Verification items for the finished model (mm, model axes). A direction names the side the tool comes from. Round coordinates to 2 decimals unless told otherwise and drop trailing zeros. Order: outer loops, then holes, each group sorted by start corner. A loop starts at its lowest first (then second) coordinate and runs counter-clockwise, first axis right, second up. Notation, with made-up numbers: M -5,50.25 L -1,50.25 A21 ccw -1,81.25 Z; hole C 5,35.25 d4. An arc over 180 degrees is marked long. Use CSV: the item, a comma, the result in double quotes. Start each with the question number.
Q1. Sectioned sample at A-A (z = 22.5). Enter the section's corners in (x, y).
Q2. Sectioned sample at B-B (x = 9.5). Enter the section's corners in (y, z), and give its area (3 significant figures).
Q3. Sectioned sample at C-C (x = 24.3). Enter the section's corners in (y, z).
Q4. Mould release check, pull along Y, two halves, no side actions. Record for faces 1 (the face through (-22.3, 4.78, 29.48)), 2 (the face through (8, 0, 40)), 3 (the face through (22, -1, 31)), 4 (the face through (22.3, -4.77, 29.48)): +Y half, -Y half, draft (parallel to the pull), parting line (faces both ways), or undercut.
Q5. Sectioned sample at D-D (x = 1). Enter the section's corners in (y, z).
Q6. Gauge pin test, flat ends, axial feed: pin 1 Ø4 at (y, z) = (-4.5, 12) entering from +X; pin 2 Ø8 at (x, y) = (-21.5, -7.5) entering from +Z; pin 3 Ø5 at (x, y) = (-16, 2.5) entering from +Z. Record the tip position at first contact, or that the pin passes through.
Q7. Set-up check for faces 5 (the face through (20, -0.2, 38.3)), 6 (the face through (22, 1, 31)), 7 (the face through (18, -8, 38)), 8 (the face through (20, 0, 14)): record each of +Z, -Z, +X, -X, +Y, -Y from which the full face is reachable in a straight line by a thin tool's end or side.
Q8. Scan lines: line 1 (Y direction, x = -24.3, z = 29.1); line 2 (Z direction, x = 1, y = 5.75); line 3 (X direction, y = -6.25, z = 10.5). Record each from-to range of solid material in increasing order.
Autodesk Inventor part; units mm, degrees
ref_plane "Work Plane1" through (0, 0, 28.3) normal (0, 0, 1) x (1, 0, 0)
ref_plane "YZ Plane" through (0, 0, 0) normal (1, 0, 0) x (0, 1, 0)
ref_plane "XZ Plane" through (0, 0, 0) normal (0, 1, 0) x (-1, 0, 0)
sketch "Sketch1" plane through (0, 0, 0) normal (0, 0, 1) x (1, 0, 0)
  line L0 (-20, -10) -> (20, -10)
  line L1 (20, -10) -> (20, 10)
  line L2 (20, 10) -> (-20, 10)
  line L3 (-20, 10) -> (-20, -10)
  line L4 (-20, -10) -> (20, 10) construction
  line L5 (20, -10) -> (-20, 10) construction
  point P0 (0, 0)
  dimension "d0" = 40
  dimension "d1" = 20
extrude "Extrusion1" add sketch "Sketch1" along normal blind 39
ref_plane "Work Plane1" through (0, 0, 28.3) normal (0, 0, 1) x (1, 0, 0)
sketch "Sketch2" plane through (0, 0, 28.3) normal (0, 0, 1) x (1, 0, 0)
  line L0 (20, -10) -> (-20, -10)
  line L1 (-20, -10) -> (-20, 10)
  line L2 (-20, 10) -> (20, 10)
  line L3 (20, 10) -> (20, -10)
  line L4 (-27, -10) -> (27, -10)
  line L5 (27, -10) -> (27, 10)
  line L6 (27, 10) -> (-27, 10)
  line L7 (-27, 10) -> (-27, -10)
  line L8 (-27, -10) -> (27, 10) construction
  line L9 (27, -10) -> (-27, 10) construction
  line L10 (-27, -4.7082) -> (-24.3, -4.7082) construction
  line L11 (-24.3, -4.7) -> (-24.3, 4.7) construction
  arc A0 (-26.154, 3.95) -> (-26.154, 5.45) centre (-24.3, 4.7) ccw
  arc A1 (-26.1507, -5.4582) -> (-26.1573, -3.9582) centre (-24.3, -4.7) ccw
  line L12 (0, 13.3238) -> (0, -12.3222) construction
  arc A2 (26.154, 5.45) -> (26.154, 3.95) centre (24.3, 4.7) ccw
  arc A3 (26.1573, -3.9582) -> (26.1507, -5.4582) centre (24.3, -4.7) ccw
  line L13 (-27, 3.95) -> (-27, 5.45)
  line L14 (-27, -5.4582) -> (-27, -3.9582)
  line L15 (-27, 5.45) -> (-26.154, 5.45)
  line L16 (-27, 3.95) -> (-26.154, 3.95)
  line L17 (-27, -3.9582) -> (-26.1573, -3.9582)
  line L18 (-27, -5.4582) -> (-26.1507, -5.4582)
  line L19 (27, 5.45) -> (26.154, 5.45)
  line L20 (27, 3.95) -> (26.154, 3.95)
  line L21 (27, -3.9582) -> (26.1573, -3.9582)
  line L22 (27, -5.4582) -> (26.1507, -5.4582)
  point P0 (0, 0)
  point P1 (24.3, -4.7082)
  point P2 (-27, 4.7)
  dimension "d5" = 54
  dimension "d13" = 2.7
  dimension "d14" = 9.4
  dimension "furos" = 4
  dimension "d16" = 4
  dimension "d29" = 1.5
  dimension "d30" = 1.5
extrude "Extrusion2" add sketch "Sketch2" along normal blind 2.4 contours L3 L6 L5 L19 A2 L20 L21 A3 L22 L4 | L4 L7 L18 A1 L17 L16 A0 L15 L6 L1 | L22 A3 L21 L5 | L7 L17 A1 L18 | L5 L20 A2 L19 | L15 A0 L16 L7
sketch "Sketch3" plane through (0, 0, 0) normal (0, 1, 0) x (-1, 0, 0)
  line L0 (-27, 28.3) -> (-27, 30.7)
  line L1 (-27, 30.7) -> (-20, 30.7)
  line L2 (-20, 30.7) -> (-20, 39)
  line L3 (-20, 39) -> (20, 39)
  line L4 (20, 39) -> (20, 30.7)
  line L5 (20, 30.7) -> (27, 30.7)
  line L6 (27, 30.7) -> (27, 28.3)
  line L7 (27, 28.3) -> (20, 28.3)
  line L8 (20, 28.3) -> (20, 0)
  line L9 (20, 0) -> (-20, 0)
  line L10 (-20, 0) -> (-20, 28.3)
  line L11 (-20, 28.3) -> (-27, 28.3)
  line L12 (20, 30.7) -> (20, 33.2)
  line L13 (20, 33.2) -> (27, 30.7)
  line L14 (27, 30.7) -> (20, 30.7)
  line L15 (0, 28.3) -> (0, 40.3429)
  line L16 (-20, 39) -> (-20, 30.7)
  line L17 (-20, 30.7) -> (-27, 30.7)
  line L18 (-20, 30.7) -> (-20, 33.2)
  line L19 (-20, 33.2) -> (-27, 30.7)
  line L20 (-27, 30.7) -> (-20, 30.7)
  point P0 (0, 0)
  dimension "d8" = 2.5
extrude "Extrusion4" add sketch "Sketch3" along normal mid plane 2 contours L19 L2 L1 | L13 L5 L4
extrude "Extrusion5" cut sketch "Sketch2" along normal up to surface (2.4 mm away) contours L22 A3 L21 L5 | L7 L17 A1 L18 | L5 L20 A2 L19 | L15 A0 L16 L7
sketch "Sketch4" plane through (0, 0, 39) normal (0, 0, 1) x (1, 0, 0)
  line L0 (20, 10) -> (20, -10) construction
  line L1 (20, 0) -> (9.5, 0) construction
  circle A0 centre (9.5, 0) radius 1.5
  point P0 (0, 0)
  dimension "d19" = 10.5
  dimension "d20" = 3
extrude "Extrusion6" add sketch "Sketch4" along normal blind 1.5
sketch "Sketch5" plane through (9.5, 0, 40.5) normal (0, 0, 1) x (1, 0, 0)
  circle A0 centre (0, 0) radius 3
  point P0 (-9.5, 0)
  dimension "d23" = 6
extrude "Extrusion7" add sketch "Sketch5" along normal blind 3
sketch "Sketch6" plane through (0, 0, 39) normal (0, 0, 1) x (1, 0, 0)
  circle A0 centre (9.5, 0) radius 1.5
  line L0 (20, 10) -> (20, -10)
  line L1 (20, -10) -> (-20, -10)
  line L2 (-20, -10) -> (-20, 10)
  line L3 (-20, 10) -> (20, 10)
  line L4 (-20, 10) -> (-15, 10)
  line L5 (-15, 10) -> (-15, -10)
  line L6 (-15, -10) -> (-20, -10)
  line L7 (-20, -10) -> (-20, 10)
  arc A1 (12.7016, -10) -> (12.7016, 10) centre (9.5, 0) ccw
  point P0 (0, 0)
  point P1 (20, 0)
  dimension "d26" = 5
extrude "Extrusion8" cut sketch "Sketch6" against normal blind 1 contours L0 A1 L3 | L0 L1 A1 | L5 L1 L2 L3
fillet "Fillet1" radius 2 4 edges at (-27, -10, 29.5) (-27, 10, 29.5) (27, -10, 29.5) (27, 10, 29.5)
fillet "Fillet2" radius 0.5 15 edges at (-1.1492, -10, 39) (20, 0, 39) (-1.1492, 10, 39) (-15, 0, 39) (-17.5, -10, 38) (-20, 0, 38) (-17.5, 10, 38) (20, 10, 34.35) (20, -10, 34.35) (20, -10, 14.15) (20, 10, 14.15) (-20, -10, 14.15) (-20, -10, 34.35) (-20, 10, 34.35) (-20, 10, 14.15)
equation "\"d16\" = furos"
properties part number "Servo996R_180º"
Verdict:
1,outline,"M -20,-9.5 A0.5 ccw -19.5,-10 L 19.5,-10 A0.5 ccw 20,-9.5 L 20,9.5 A0.5 ccw 19.5,10 L -19.5,10 A0.5 ccw -20,9.5 Z"
2,outline,"M -10,0 L 10,0 L 10,38.5 A0.5 ccw 9.5,39 L 1.5,39 L 1.5,40.5 L 3,40.5 L 3,43.5 L -3,43.5 L -3,40.5 L -1.5,40.5 L -1.5,39 L -9.5,39 A0.5 ccw -10,38.5 Z"
2,area,"802 mm²"
3,outline,"M -10,28.3 L -6.7,28.3 L -6.7,30.7 L -10,30.7 Z; M -2.7,28.3 L 2.7,28.3 L 2.7,30.7 L 1,30.7 L 1,31.66 L -1,31.66 L -1,30.7 L -2.7,30.7 Z; M 6.7,28.3 L 10,28.3 L 10,30.7 L 6.7,30.7 Z"
4,face 1,"undercut"
4,face 2,"parting line"
4,face 3,"-Y half"
4,face 4,"undercut"
5,outline,"M -10,0 L 10,0 L 10,38.5 A0.5 ccw 9.5,39 L -9.5,39 A0.5 ccw -10,38.5 Z"
6,pin 1,"stops at x = 20"
6,pin 2,"stops at z = 38"
6,pin 3,"stops at z = 39"
7,face 5,"+Z, +X"
7,face 6,"+Z, +X, +Y"
7,face 7,"+Z, +X, -Y"
7,face 8,"-Z, +X, +Y, -Y"
8,line 1,"y = -10 to -6.7, -2.7 to 2.7, 6.7 to 10"
8,line 2,"z = 0 to 39"
8,line 3,"x = -20 to 20"
